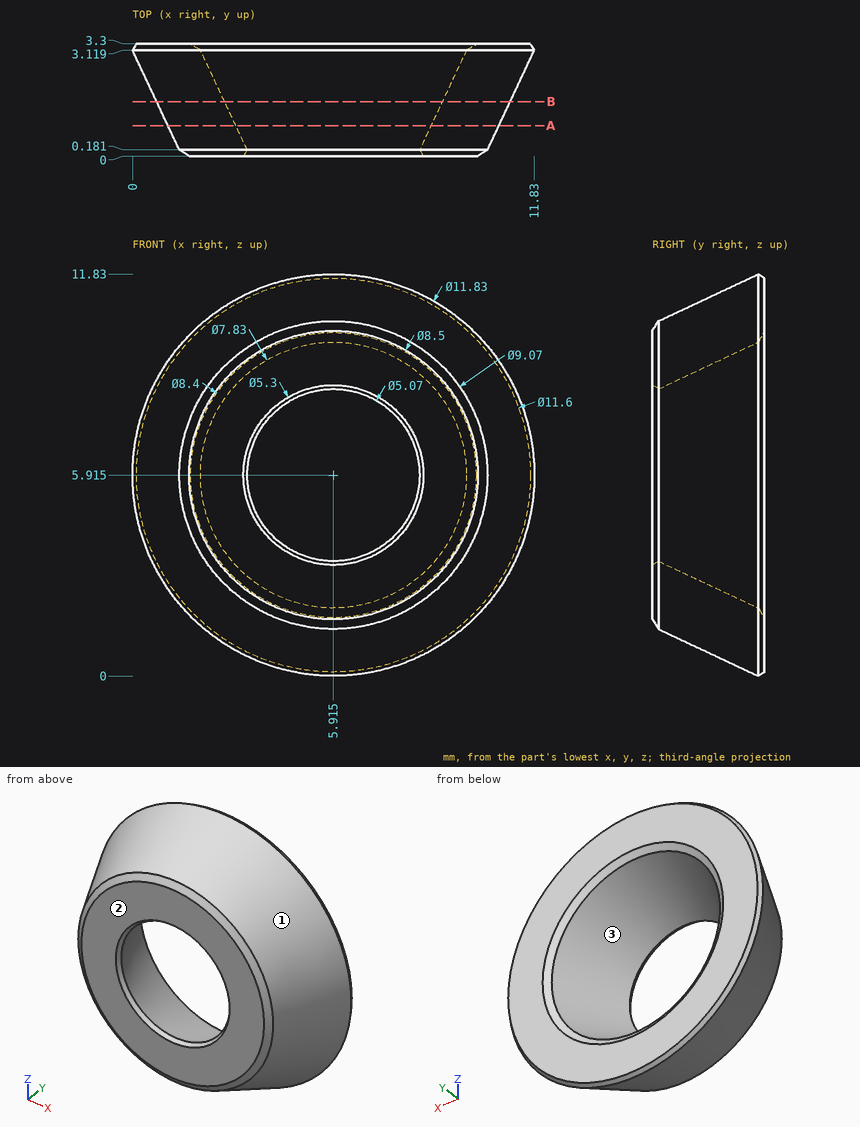
Input: dimensioned drawing with shaded views. Units: mm. Origin: part minimum x, y, z. Round coordinates to 2 decimals unless told otherwise and drop trailing zeros. Order: outer loops, then holes, each group sorted by start corner. A loop starts at its lowest first (then second) coordinate and runs counter-clockwise, first axis right, second up. Notation, with made-up numbers: M 10.5,-31 L 14.5,-31 A15 cw 14.5,-6 Z; hole C 89.25,19.5 d9. An arc over 180 degrees is marked long. Use one line per item in the form item = value. Start each with the question number.
Q1. Pin query (flat end, axial travel): pin 1 Ø1 at (y, z) = (2, 10) entering from -X; pin 2 Ø1 at (x, z) = (7, 8) entering from -Y. Return the tip coordinate at first contact, or that it passes through.
Q2. Mould query, pull axis X, two halves, no side actions, for the marked faces 1, 2 and 3. Classes: +X half, -X half, draft (parallel to the pull), parting line (faces both ways), or undercut.
Q3. Material intervals for line 1 (Z direction, x = 4.5, y = 0.65) (1 decimal); line 2 (Z direction, x = 5.25, y = 2.4); line 3 (X direction, y = 1.3, z = 3.25), sorted ascending. Write a range as [from, to].
Q4. Cut plane A-A (y = 0.9). Return loops of the section in (x, z) (1 decimal), and give its area (3 significant figures).
Q5. Cut plane B-B (y = 1.6). Return loops of the section in (x, z) (1 decimal), and give its area (3 significant figures).
Geometry results:
q1.pin_1 = 1.79
q1.pin_2 = 0
q2.face_1 = parting line
q2.face_2 = draft
q2.face_3 = undercut
q3.line_1 = [1.4, 3.6], [8.3, 10.5]
q3.line_2 = [0.38, 2.4], [9.43, 11.45]
q3.line_3 = [1.61, 4.41], [7.42, 10.22]
q4.outline = C 5.9,5.9 d9.7; hole C 5.9,5.9 d5.7
q4.area = 48.7 mm^2
q5.outline = C 5.9,5.9 d10.4; hole C 5.9,5.9 d6.4
q5.area = 52.8 mm^2
